```python
from build123d import *

# Parameters (mm, degrees)
BASE_FLANGE1_DEPTH            = 1365.25
EDGE_FLANGE1_STRIP_W          = 19.812
EDGE_FLANGE1_STRIP_H          = 3.175
EDGE_FLANGE1_STRIP_CUT_DEPTH  = 25.4
EDGE_FLANGE1_RELIEF_W         = 21.3995
EDGE_FLANGE1_RELIEF_H         = 1.5875
EDGE_FLANGE1_RELIEF_CUT_DEPTH = 3.175
EDGE_FLANGE1_DEPTH            = 25.4


# Sheet-metal steps are written as plain solids
with BuildPart() as part:
    # Sketch1 → Base-Flange1 (new body)
    with BuildSketch(Plane.XY):
        with BuildLine():
            Line((0, 120.65), (0, 6.35))
            ThreePointArc((0, 6.35), (1.859871939, 1.859871939), (6.35, 0))
            Line((6.35, 0), (79.375, 0))
            ThreePointArc((79.375, 0), (83.865128061, 1.859871939), (85.725, 6.35))
            Line((85.725, 6.35), (85.725, 25.4))
            Line((85.725, 25.4), (82.55, 25.4))
            Line((82.55, 25.4), (82.55, 6.35))
            ThreePointArc((82.55, 6.35), (81.62006403, 4.10493597), (79.375, 3.175))
            Line((79.375, 3.175), (6.35, 3.175))
            ThreePointArc((6.35, 3.175), (4.10493597, 4.10493597), (3.175, 6.35))
            Line((3.175, 6.35), (3.175, 120.65))
            Line((3.175, 120.65), (0, 120.65))
        make_face()
    extrude(amount=BASE_FLANGE1_DEPTH)

    # Edge-Flange1 strip (across the edge) → Edge-Flange1 strip cut (cut)
    with BuildSketch(Plane(origin=(31.75, 3.175, 1364.488), x_dir=(0, 0, -1), z_dir=(1, 0, 0))):
        with Locations((-3.556, -1.5875)):
            Rectangle(EDGE_FLANGE1_STRIP_W, EDGE_FLANGE1_STRIP_H)
    extrude(amount=EDGE_FLANGE1_STRIP_CUT_DEPTH, mode=Mode.SUBTRACT)

    # Edge-Flange1 relief (on the sheet) → Edge-Flange1 relief cut (cut)
    with BuildSketch(Plane(origin=(31.75, 3.175, 1358.138), x_dir=(0, 0, -1), z_dir=(0, 1, 0))):
        with Locations((-9.11225, 0.79375)):
            Rectangle(EDGE_FLANGE1_RELIEF_W, EDGE_FLANGE1_RELIEF_H)
        with Locations((-9.11225, -26.19375)):
            Rectangle(EDGE_FLANGE1_RELIEF_W, EDGE_FLANGE1_RELIEF_H)
    extrude(amount=-EDGE_FLANGE1_RELIEF_CUT_DEPTH, mode=Mode.SUBTRACT)

    # Edge-Flange1 section (across the edge) → Edge-Flange1 (add)
    with BuildSketch(Plane(origin=(31.75, 3.175, 1364.488), x_dir=(0, 0, -1), z_dir=(1, 0, 0))):
        with BuildLine():
            Line((0, 3.175), (0, 22.225))
            Line((0, 22.225), (3.175, 22.225))
            Line((3.175, 22.225), (3.175, 3.175))
            ThreePointArc((3.175, 3.175), (4.10493597, 0.92993597), (6.35, 0))
            Line((6.35, 0), (6.35, -3.175))
            ThreePointArc((6.35, -3.175), (1.859871939, -1.315128061), (0, 3.175))
        make_face()
    extrude(amount=EDGE_FLANGE1_DEPTH)


solid = part.part
```
The listing builds one solid part. Answer for the finished solid, in the listing's coordinates (mm). A direction names the side the tool comes from. Coordinates: 2 decimals unless noted, no trailing zeros. Write each loop counter-clockwise with the first axis right and the second up, starting at its lowest first coordinate (ties: lowest second). Pieces come first, ordered by that corner, then holes.
Q1. Section B-B, the plane z = 242 is taken. Write down the section's boundary in (x, y) (3 decimals), then the cut area to 3 significant figures.
Returned:
outline: (0, 6.35) arc R6.35 ccw to (6.35, 0) - (79.375, 0) arc R6.35 ccw to (85.725, 6.35) - (85.725, 25.4) - (82.55, 25.4) - (82.55, 6.35) arc R3.175 cw to (79.375, 3.175) - (6.35, 3.175) arc R3.175 cw to (3.175, 6.35) - (3.175, 120.65) - (0, 120.65) - close
area: 703 mm2
Q2. The mould has two halves that part along X. Classify faces 1 (the flat face through (0, 64, 673)), 2 (the flat face through (3.175, 63, 673)), 3 (the flat face through (1, 29, 0)): released by +X, released by -X, zero draft, split by the parting line, or undercut.
Returned:
face 1: released by -X
face 2: undercut
face 3: zero draft
Q3. Section A-A, the plane x = 44.5 is taken. Write down the section's boundary in (y, z) (3 decimals).
Returned:
outline: (0, 0) - (3.175, 0) - (3.175, 1358.138) arc R3.175 cw to (6.35, 1361.313) - (25.4, 1361.313) - (25.4, 1364.488) - (6.35, 1364.488) arc R6.35 ccw to (0, 1358.138) - close
Q4. Find the intervals of material crossed by line 1 along X through (y, z) = (9, 1211) (3 decimals); line 2 along Y through (x, z) = (16, 1171.5) (3 decimals), in increasing order.
Returned:
line 1: x = 0 to 3.175, 82.55 to 85.725
line 2: y = 0 to 3.175
Q5. Which of the six approach directions +Z, -Z, +X, -X, +Y, -Y give full straight-line access (tool end or side, diameter ignored) to faces 4 (the flat face through (3, 47, 1365.25)), 5 (the flat face through (43, 3.175, 673))?
Returned:
face 4: +Z, +X, -X, +Y, -Y
face 5: -Z, +Y
Q6. Given P1, Ø15, axis at x = 42, y = 12.5, coming from the +Z side; P2, Ø22, axis at x = 57.5, z = 541.5, coming from the +Y side (3 decimals); P3, Ø1, axis at x = 38.5, z = 1362.5, coming from the +Y side, each flat-ended and moving along its own axis, determine where each tip first touches the part or whether it passes through.
Returned:
P1: stops at z = 1364.49
P2: stops at y = 3.175
P3: stops at y = 25.4
Q7. Section C-C, the plane y = 44 is taken. Write down the section's boundary in (x, z) (3 decimals), then the cut area to 3 significant figures.
Returned:
outline: (0, 0) - (3.175, 0) - (3.175, 1365.25) - (0, 1365.25) - close
area: 4,330 mm2
